Verification items for the finished model (mm, model axes). A direction names the side the tool comes from. Give positions to 0.01 mm unless a question says otherwise; leave off trailing zeros. Order: outer loops, then holes, each group sorted by start corner. A loop starts at its lowest first (then second) coordinate and runs counter-clockwise, first axis right, second up. Notation, with made-up numbers: (37.5, 29) -> (94.5, 29) arc R16 cw to (94.5, 51) -> close; hole circle Ø6 at (41.25, 46.5). An arc over 180 degrees is marked (long way). Return JSON: item names as keys, results as strings. Group by question number.
(1) Cross-section at C-C on z = 44.5. Enter the section's corners in (x, y).
(2) Tool access check on faces 1 (the face through (5.13, -14.52, 11.29)), 2 (the face through (-14.985, 11.652, 33.199)). Record the directions out of +Z, -Z, +X, -X, +Y, -Y that give a thin tool (end or side, any length) a straight path to the whole face; none if there is none.
(3) Cross-section at A-A on y = 17. Enter the section's corners in (x, z).
(4) Depth check by flat-ended pin: pin 1 Ø12 at (x, z) = (-2.5, 8) entering from +Y; pin 2 Ø4 at (x, z) = (15.5, 12.5) entering from +Y; pin 3 Ø2 at (y, z) = (0.5, 17) entering from -X. Enter the tip coordinate at first touch or a pass-through.
(5) Thickness scan on line 1 along Y through (x, z) = (0, 21); line 2 along Z through (x, y) = (-36.5, 2.5); line 3 along Y through (x, z) = (7, 23). Record the ranges inside material, lowest first.
(6) Release check for a two-part mould opening along X. For faces 3 (the face through (-39.742, 10.306, 5.916)), 4 (the face through (12, 12, 0)), 5 (the face through (45.296, 13.621, 5.916)), 6 (the face through (-2.367, 0.334, 27.115)) record: pulls with the +X half, pulls with the -X half, needs draft (parallel to the pull), parting line crosses it, or undercut.
(7) Cross-section at B-B on y = 8.5. Enter the section's corners in (x, z), then the cut area to 3 significant figures.
from build123d import *

# Parameters (mm, degrees)
F0_R     = 15
F1_DEPTH = 12
F0_R_2   = 10.918635
F2_DEPTH = 55
F3_R     = 2.5


with BuildPart() as f1:
    # F0 (on Top) → F1 (new body)
    with BuildSketch(Plane.XY):
        Polygon((43.459415, 41.090946), (-41.540585, 37.36122), (-37.89244, -17.517657), (47.082786, -13.090479), align=None)
        with Locations((0, 10.992759)):
            Circle(F0_R, mode=Mode.SUBTRACT)
    extrude(amount=F1_DEPTH)

    # F0 (on Top) → F2 (join)
    with BuildSketch(Plane.XY):
        with Locations((0, 10.992759)):
            Circle(F0_R)
        with Locations((0, 10.992759)):
            Circle(F0_R_2, mode=Mode.SUBTRACT)
    extrude(amount=F2_DEPTH)

    # F3
    f3_edges = [f1.edges().sort_by_distance(p)[0] for p in [
        (4.595173, -15.304068, 12),
    ]]
    fillet(f3_edges, radius=F3_R)


solid = f1.part
Verdict:
{
 "1": {"outline": "circle Ø30 at (0, 10.99); hole circle Ø21.84 at (0, 10.99)"},
 "2": {"face 1": "+Z, +X, -Y", "face 2": "+Z"},
 "3": {"outline": "(-40.19, 0) -> (-9.12, 0) -> (-9.12, 55) -> (-13.74, 55) -> (-13.74, 12) -> (-40.19, 12) -> close; (9.12, 0) -> (45.07, 0) -> (45.07, 12) -> (13.74, 12) -> (13.74, 55) -> (9.12, 55) -> close"},
 "4": {"pin 1": "y = 39.34", "pin 2": "y = 39.95", "pin 3": "x = -11.61"},
 "5": {"line 1": "-4.01 to 0.07, 21.91 to 25.99", "line 2": "0 to 12", "line 3": "-2.27 to 2.61, 19.37 to 24.26"},
 "6": {"face 3": "pulls with the -X half", "face 4": "needs draft", "face 5": "pulls with the +X half", "face 6": "undercut"},
 "7": {"outline": "(-39.62, 0) -> (-10.63, 0) -> (-10.63, 55) -> (-14.79, 55) -> (-14.79, 12) -> (-39.62, 12) -> close; (10.63, 0) -> (45.64, 0) -> (45.64, 12) -> (14.79, 12) -> (14.79, 55) -> (10.63, 55) -> close", "area": "1,130 mm²"}
}
